```python
from build123d import *

# Parameters (mm, degrees)
SKETCH1_R                       = 5.08
BOSS_EXTRUDE1_DEPTH             = 6.35
SKETCH2_R                       = 4.2672
BOSS_EXTRUDE2_DEPTH             = 12.7
F_21_0_159_DIAMETER_HOLE1_D     = 3.999999874
F_21_0_159_DIAMETER_HOLE1_DEPTH = 12.7


with BuildPart() as part:
    # Sketch1 → Boss-Extrude1 (new body)
    with BuildSketch(Plane(origin=(0, 0, 0), x_dir=(0, 0, -1), z_dir=(1, 0, 0))):
        Circle(SKETCH1_R)
    extrude(amount=BOSS_EXTRUDE1_DEPTH)

    # Sketch2 → Boss-Extrude2 (add)
    with BuildSketch(Plane.ZY):
        with Locations(Location((0, 0, 0), (0, 0, 180))):
            Circle(SKETCH2_R)
    extrude(amount=BOSS_EXTRUDE2_DEPTH)

    # #21 (0.159) Diameter Hole1
    with Locations(Plane.ZY.offset(12.7)):
        with Locations((0, 0)):
            Hole(F_21_0_159_DIAMETER_HOLE1_D / 2, depth=F_21_0_159_DIAMETER_HOLE1_DEPTH)


solid = part.part
```
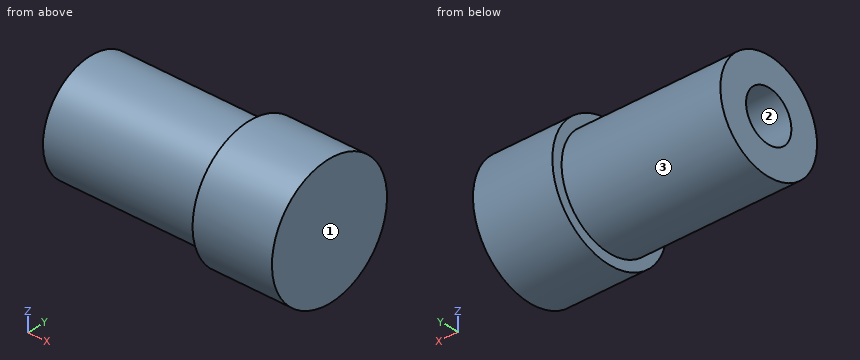
CAD build for the part. Positions are in the model's coordinates, mm. Face numbers are marked on the shaded views. Round coordinates to 2 decimals unless told otherwise and drop trailing zeros. Write each loop counter-clockwise with the first axis right and the second up, starting at its lowest first coordinate (ties: lowest second). Pieces come first, ordered by that corner, then holes. Notation, with made-up numbers: (-33, 10.25) -> (18, 10.25) arc R24 cw to (18, 44.25) -> close; hole circle Ø2 at (19, 75.25). An arc over 180 degrees is marked (long way). Answer in a Markdown table with one row per item. Add a question column.
Item 1: Mould opens along Y. For the marked faces 1, 2 and 3 say: pulls with the +Y half, pulls with the -Y half, needs draft (parallel to the pull), parting line crosses it, or undercut.
Item 2: Drop flat-ended pins along their axis: pin 1 Ø3 at (y, z) = (0, 0) entering from -X; pin 2 Ø5 at (y, z) = (0.5, -1.5) entering from -X; pin 3 Ø1 at (x, y) = (-3, 1) entering from +Z; pin 4 Ø1.5 at (x, z) = (-3.5, 0.5) entering from +Y. Give the stop position or say it passes through.
Item 3: Saw through at D-D, the plane x = 1. Write the cut outline in (y, z).
Item 4: Saw through at C-C, the plane x = -7.75. Write the cut outline in (y, z).
Item 5: Drill centre lines: line 1 (Y direction, x = -5, z = 0); line 2 (X direction, y = 0.75, z = 4.5); line 3 (Z direction, x = -7.5, y = 0.25). Where is each one in solid material? Low to high. Write a range as from..to.
Item 6: Saw through at A-A, the plane y = 0. Write the cut outline in (x, z).
Findings below:
| question | item | result |
|---|---|---|
| 1 | face 1 | needs draft |
| 1 | face 2 | undercut |
| 1 | face 3 | parting line crosses it |
| 2 | pin 1 | stops at x = 0 |
| 2 | pin 2 | stops at x = -12.7 |
| 2 | pin 3 | stops at z = 4.24 |
| 2 | pin 4 | stops at y = 4.27 |
| 3 | outline | circle Ø10.16 at (0, 0) |
| 4 | outline | circle Ø8.53 at (0, 0); hole circle Ø4 at (0, 0) |
| 5 | line 1 | y = -4.27..-2, 2..4.27 |
| 5 | line 2 | x = 0..6.35 |
| 5 | line 3 | z = -4.26..-1.98, 1.98..4.26 |
| 6 | outline | (-12.7, -4.27) -> (0, -4.27) -> (0, -5.08) -> (6.35, -5.08) -> (6.35, 5.08) -> (0, 5.08) -> (0, 4.27) -> (-12.7, 4.27) -> (-12.7, 2) -> (0, 2) -> (0, -2) -> (-12.7, -2) -> close |
